```python
from build123d import *

# Parameters (mm, degrees)
F0_W          = 20.5
F0_H          = 42
F1_DEPTH      = 39.5
F2_START      = 8.5
F2_DEPTH      = 2.5
F5_W          = 6.5
F5_H          = 5
F6_DEPTH      = 8
F7_SIZE2      = 4.5
F7_SIZE       = 7.5
F8_R          = 4
F9_DEPTH      = 1
F9_DEPTH_BACK = 3.5
F10_ANGLE     = 180
F12_ANGLE     = -90


# Not quite as in the source:
# - a feature names something its author has since deleted; it is built from what else it names


with BuildPart() as f1:
    # F0 (on Top) → F1 (new body)
    with BuildSketch(Plane.XY):
        with Locations((0, -10.5)):
            Rectangle(F0_W, F0_H)
    extrude(amount=F1_DEPTH)

    # F0 (on Top) → F2 (join)
    with BuildSketch(Plane.XY.offset(F2_START)):
        with BuildLine():
            Line((-10.25, 10.5), (10.25, 10.5))
            Line((10.25, 10.5), (10.25, 17.5))
            Line((10.25, 17.5), (6.2807764064, 17.5))
            ThreePointArc((6.2807764064, 17.5), (5.25, 13.25), (4.2192235936, 17.5))
            Line((4.2192235936, 17.5), (-4.2192235936, 17.5))
            ThreePointArc((-4.2192235936, 17.5), (-5.25, 13.25), (-6.2807764064, 17.5))
            Line((-6.2807764064, 17.5), (-10.25, 17.5))
            Line((-10.25, 17.5), (-10.25, 10.5))
        make_face()
        with BuildLine():
            Line((10.25, -38.5), (10.25, -31.5))
            Line((10.25, -31.5), (-10.25, -31.5))
            Line((-10.25, -31.5), (-10.25, -38.5))
            Line((-10.25, -38.5), (-6.2807764064, -38.5))
            ThreePointArc((-6.2807764064, -38.5), (-5.25, -34.25), (-4.2192235936, -38.5))
            Line((-4.2192235936, -38.5), (4.2192235936, -38.5))
            ThreePointArc((4.2192235936, -38.5), (5.25, -34.25), (6.2807764064, -38.5))
            Line((6.2807764064, -38.5), (10.25, -38.5))
        make_face()
    extrude(amount=F2_DEPTH)

    # F3 (on Right) → F4 (revolve)
    with BuildSketch(Plane.YZ):
        Polygon((5.5, -2), (7, 0), (0, 0), (0, -6), (3, -6), (3, -2), align=None)
    revolve(axis=Axis((0, 0, -3), (0, 0, 1)))

    # F5 (on face) → F6 (join)
    with BuildSketch(Plane(origin=(0, 10.5, 0), x_dir=(-1, 0, 0), z_dir=(0, 1, 0))):
        with Locations((0, 33)):
            Rectangle(F5_W, F5_H)
    extrude(amount=F6_DEPTH)

    # F7
    f7_edges = [f1.edges().sort_by_distance(p)[0] for p in [
        (0, -31.5, 0),
    ]]
    f7_side = f1.faces().sort_by_distance((0, -12.786008, 0))[0]
    chamfer(f7_edges, length=F7_SIZE, length2=F7_SIZE2, reference=f7_side)

    # F8 (on face) → F9 (join, two sides)
    with BuildSketch(Plane(origin=(0, 0, 8.5), x_dir=(1, 0, 0), z_dir=(0, 0, -1))) as f9_sk:
        with Locations((-5.25, 36.5)):
            Circle(F8_R)
        with Locations((5.25, 36.5)):
            Circle(F8_R)
        with BuildLine():
            Line((4.2192235936, -17.5), (1.7858983849, -17.5))
            ThreePointArc((1.7858983849, -17.5), (5.25, -19.5), (8.7141016151, -17.5))
            Line((8.7141016151, -17.5), (6.2807764064, -17.5))
            ThreePointArc((6.2807764064, -17.5), (5.25, -13.25), (4.2192235936, -17.5))
        make_face()
        with BuildLine():
            Line((-8.7141016151, -17.5), (-6.2807764064, -17.5))
            ThreePointArc((-6.2807764064, -17.5), (-5.25, -13.25), (-4.2192235936, -17.5))
            Line((-4.2192235936, -17.5), (-1.7858983849, -17.5))
            ThreePointArc((-1.7858983849, -17.5), (-1.3862966948, -16.5352761804), (-1.25, -15.5))
            ThreePointArc((-1.25, -15.5), (-6.2852761804, -11.6362966948), (-8.7141016151, -17.5))
        make_face()
        with BuildLine():
            ThreePointArc((-4.2192235936, -17.5), (-5.25, -13.25), (-6.2807764064, -17.5))
            Line((-6.2807764064, -17.5), (-8.7141016151, -17.5))
            ThreePointArc((-8.7141016151, -17.5), (-5.25, -19.5), (-1.7858983849, -17.5))
            Line((-1.7858983849, -17.5), (-4.2192235936, -17.5))
        make_face()
        with BuildLine():
            ThreePointArc((9.25, -15.5), (4.2147238196, -11.6362966948), (1.7858983849, -17.5))
            Line((1.7858983849, -17.5), (4.2192235936, -17.5))
            ThreePointArc((4.2192235936, -17.5), (5.25, -13.25), (6.2807764064, -17.5))
            Line((6.2807764064, -17.5), (8.7141016151, -17.5))
            ThreePointArc((8.7141016151, -17.5), (9.1137033052, -16.5352761804), (9.25, -15.5))
        make_face()
    extrude(amount=F9_DEPTH)
    extrude(f9_sk.sketch, amount=-F9_DEPTH_BACK)


with BuildPart() as f1_1:
    # F10: moved
    add(f1.part.rotate(Axis((0, 5.25, 0), (0, 1, 0)), F10_ANGLE))


with BuildPart() as f1_2:
    # F11: moved
    add(f1_1.part.moved(Location((0, 0, -6))))


with BuildPart() as f1_3:
    # F12: moved
    add(f1_2.part.rotate(Axis((0, 0, -3), (0, 0, 1)), F12_ANGLE))


solid = f1_3.part
```
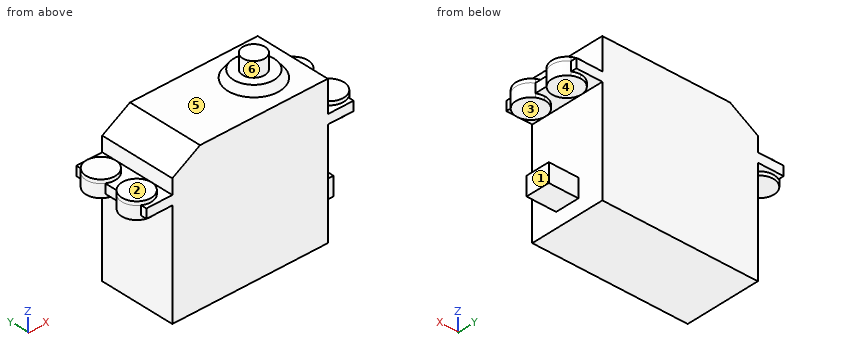
The listing builds one solid part. Answer for the finished solid, in the listing's coordinates (mm). Face numbers are marked on the shaded views. A direction names the side the tool comes from. Coordinates: 2 decimals unless noted, no trailing zeros. Write each loop counter-clockwise with the first axis right and the second up, starting at its lowest first coordinate (ties: lowest second). Pieces come first, ordered by that corner, then holes.
Q1. Find the intervals of material crossed by line 1 along Z through (x, y) = (16, -0.75); line 2 along Z through (x, y) = (-12, -5.75); line 3 along X through (y, z) = (-0.25, -20), in increasing order.
Returned:
line 1: z = -41.5 to -36.5, -17 to -14.5
line 2: z = -45.5 to -6
line 3: x = -31.5 to 10.5
Q2. Section B-B, the plane y = 0 is taken. Write down the section's boundary in (x, z).
Returned:
outline: (-38.5, -17) - (-31.5, -17) - (-31.5, -45.5) - (10.5, -45.5) - (10.5, -41.5) - (18.5, -41.5) - (18.5, -36.5) - (10.5, -36.5) - (10.5, -17) - (17.5, -17) - (17.5, -14.5) - (10.5, -14.5) - (10.5, -6) - (7, -6) - (5.5, -4) - (3, -4) - (3, 0) - (-3, 0) - (-3, -4) - (-5.5, -4) - (-7, -6) - (-24, -6) - (-31.5, -10.5) - (-31.5, -14.5) - (-38.5, -14.5) - close
Q3. The mould has two halves that part along Z. Classify the marked faces 4, 5 and 6: released by +Z, released by -Z, zero draft, split by the parting line, or undercut.
Returned:
face 4: undercut
face 5: released by +Z
face 6: zero draft
Q4. Section C-C, the plane z = -40 is taken. Write down the section's boundary in (x, y), then the cut area to 3 significant figures.
Returned:
outline: (-31.5, -10.25) - (10.5, -10.25) - (10.5, -3.25) - (18.5, -3.25) - (18.5, 3.25) - (10.5, 3.25) - (10.5, 10.25) - (-31.5, 10.25) - close
area: 913 mm2
Q5. Given P1, Ø1.2, axis at y = 10, z = -15.5, coming from the +X side; P2, Ø5, axis at x = -24.5, y = 1.5, coming from the +Z side; P3, Ø5.5, axis at x = 15, y = -4.5, coming from the -Z side; P4, Ø4, axis at y = -4, z = -19.5, coming from the -X side, each flat-ended and moving along its own axis, determine where each tip first touches the part or whether it passes through.
Returned:
P1: stops at x = 17.5
P2: stops at z = -6
P3: stops at z = -41.5
P4: stops at x = -40.5
Q6. Section D-D, the plane x = 0 is taken. Write down the section's boundary in (y, z).
Returned:
outline: (-10.25, -45.5) - (10.25, -45.5) - (10.25, -6) - (7, -6) - (5.5, -4) - (3, -4) - (3, 0) - (-3, 0) - (-3, -4) - (-5.5, -4) - (-7, -6) - (-10.25, -6) - close
Q7. Section A-A, the plane x = -36.5 is taken. Write down the section's boundary in (y, z), then the cut area to 4 significant figures.
Returned:
outline: (-10.25, -17) - (-9.25, -17) - (-9.25, -18) - (-1.25, -18) - (-1.25, -17) - (1.25, -17) - (1.25, -18) - (9.25, -18) - (9.25, -17) - (10.25, -17) - (10.25, -14.5) - (9.25, -14.5) - (9.25, -13.5) - (1.25, -13.5) - (1.25, -14.5) - (-1.25, -14.5) - (-1.25, -13.5) - (-9.25, -13.5) - (-9.25, -14.5) - (-10.25, -14.5) - close
area: 83.25 mm2
Q8. Which of the six approach directions +Z, -Z, +X, -X, +Y, -Y give full straight-line access (tool end or side, diameter ignored) to the marked faces 1, 2 and 3?
Returned:
face 1: -Z, +X, +Y, -Y
face 2: +Z, -X, +Y, -Y
face 3: +X, +Y, -Y
